Can you work these out from the model? Positions are in its coordinate system, mm. Face numbers are marked on the shaded views. Round coordinates to 2 decimals unless told otherwise and drop trailing zeros. Order: outer loops, then holes, each group sorted by start corner. A loop starts at its lowest first (then second) coordinate and runs counter-clockwise, first axis right, second up. Notation, with made-up numbers: (-21.75, 72) - (14.25, 72) arc R23 cw to (14.25, 110) - close; hole circle Ø11 at (50.5, 10). An arc over 180 degrees is marked (long way). Write item = value, one per line.
Autodesk Inventor part; units mm, degrees
ref_plane "YZ Plane" through (0, 0, 0) normal (1, 0, 0) x (0, 1, 0)
ref_plane "XZ Plane" through (0, 0, 0) normal (0, 1, 0) x (-1, 0, 0)
ref_plane "XY Plane" through (0, 0, 0) normal (0, 0, 1) x (1, 0, 0)
sketch "Sketch1" plane through (0, 0, 0) normal (1, 0, 0) x (0, 1, 0)
  circle A0 centre (0, 0) radius 1.7526
  circle A1 centre (0, 0) radius 3.175
  circle A2 centre (2.0674, 6.004) radius 3.5 construction
  circle A3 centre (2.0674, 6.004) radius 1.5
  circle A4 centre (2.0674, 6.004) radius 2.5
  line L0 (-2.8751, 1.3469) -> (-0.1965, 7.0646)
  line L1 (0, 0) -> (15.875, 1.6685) construction
  line L2 (0, 0) -> (3.175, 0) construction
  line L3 (3.0949, -0.7087) -> (4.5043, 5.446)
  circle A5 centre (16.0409, 0.0897) radius 1.5875
  line L4 (15.875, 1.6685) -> (3.3375, 0.3508)
  line L5 (16.2069, -1.4891) -> (0.3319, -3.1576)
  line L6 (2.0674, 6.004) -> (0, 0) construction
  line L7 (2.0674, 6.004) -> (3.4856, 5.5157) construction
  line L8 (0, 0) -> (1.6571, -0.5706) construction
  dimension "d0" = 3.5052
  dimension "d7" = 3
  dimension "d1" = 6.35
  dimension "d4" = 7
  dimension "d8" = 5
  dimension "d9" = 6
  dimension "d10" = 15.875
  dimension "d11" = 3.175
  dimension "d15" = 6.35
  dimension "d16" = 65
extrude "Extrusion1" add sketch "Sketch1" along normal blind 3.175
fillet "Fillet1" radius 6.35 1 edges at (1.5875, 3.3375, 0.3508)
sketch "Sketch2" plane through (0, 0, 0) normal (-1, 0, 0) x (0, 0, 1)
  circle A0 centre (6.004, 2.0674) radius 1.5
  arc A1 (7.0646, -0.1965) -> (6.4319, 4.5305) centre (6.004, 2.0674) ccw
  circle A2 centre (6.004, 2.0674) radius 2.5
  point P0 (0, 0)
  point P1 (7.0646, -0.1965)
extrude "Extrusion2" add sketch "Sketch2" along normal blind 3.175
properties part number "Lever" material "Aluminum 6061"
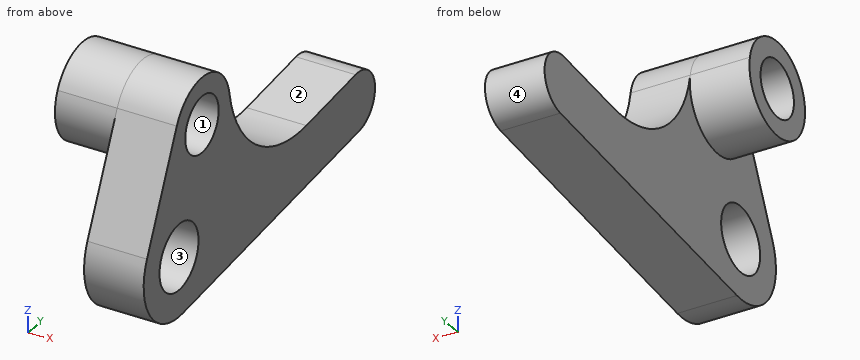
(1) If we section it at A-A (y = -1): Write out the boundary of the cut face in (x, z) (3 decimals), plus the area to 3 significant figures.
Computed:
outline = (0, -3.013) - (3.175, -3.013) - (3.175, -1.439) - (0, -1.439) - close; (0, 1.439) - (3.175, 1.439) - (3.175, 5.349) - (0, 5.349) - close
area = 17.4 mm^2
(2) If we section it at D-D (x = -1.5): Write out the boundary of the cut face in (y, z).
Computed:
outline = (-0.2, 7.06) arc R2.5 ccw (long way) to (4.53, 6.43) arc R2.5 ccw to start; hole circle Ø3 at (2.07, 6)
(3) Thinking about a two-plate mould opening in Z: for the marked faces 1, 2, 3 and 4, which applies, +Z half, -Z half, draft (parallel to the pull), parting line (faces both ways), or undercut?
Computed:
face_1 = undercut
face_2 = +Z half
face_3 = undercut
face_4 = parting line
(4) If we section it at B-B (z = -0.5): Write out the boundary of the cut face in (x, y) (3 decimals), plus the area to 3 significant figures.
Computed:
outline = (0, -3.135) - (3.175, -3.135) - (3.175, -1.68) - (0, -1.68) - close; (0, 1.68) - (3.175, 1.68) - (3.175, 17.515) - (0, 17.515) - close
area = 54.9 mm^2
(5) Will these pins go through, and if not, where does the flat tip stop? P1, Ø4.5, axis at y = 0, z = 0, coming from the -X side; P2, Ø3, axis at x = -1, y = 5, coming from the -Z side.
Computed:
P1 = 0
P2 = -2.78
(6) If we section it at C-C (x = 0.5): State how many separate pieces and enclosed holes the cut face has, plus the area to 3 significant figures.
Computed:
separate_pieces = 1
enclosed_holes = 2
area = 105 mm^2
(7) If I drill on line 1 (Y direction, x = -2.5, z = 8); line 2 (Y direction, x = 2.25, z = 5.75); line 3 (Z direction, x = 2.05, y = 0) (3 decimals), over which ranges is the centre line in solid material (lowest first)? Write a range as from..to.
Computed:
line_1 = 0.56..3.57
line_2 = -0.81..0.59, 3.55..4.69
line_3 = -3.175..-1.753, 1.753..7.41
